from build123d import *

# Parameters (mm, degrees)
SKETCH011_R      = 1
EXTRUDE013_DEPTH = 8
SKETCH009_R      = 1.2
EXTRUDE012_DEPTH = 9.3
CHAMFER001_SIZE  = 0.15
SKETCH012_R      = 0.75
EXTRUDE014_DEPTH = 2
FILLET011_R      = 0.3


with BuildPart() as extrude013:
    # Sketch011 → Extrude013 (new body)
    with BuildSketch(Plane.XY.offset(9.3)):
        with Locations((-2.5, 0)):
            Circle(SKETCH011_R)
    extrude(amount=-EXTRUDE013_DEPTH)


with BuildPart() as pinfemale002:
    # Sketch009 → Extrude012 (new body)
    with BuildSketch(Plane.XY.offset(9.6)):
        with Locations((-2.5, 0)):
            Circle(SKETCH009_R)
    extrude(amount=-EXTRUDE012_DEPTH)


with BuildPart() as pinfemale002_1:
    # Extrude012 placement: moved
    add(pinfemale002.part.moved(Location((0, 0, -0.3))))

    # Cut007: cut Extrude013
    add(extrude013.part, mode=Mode.SUBTRACT)

    # Chamfer001
    chamfer001_edges = [pinfemale002_1.edges().sort_by_distance(p)[0] for p in [
        (-3.5, 0, 9.3),
    ]]
    chamfer(chamfer001_edges, length=CHAMFER001_SIZE)


with BuildPart() as pinfemale003:
    # Sketch012 → Extrude014 (new body)
    with BuildSketch(Plane(origin=(0, 0, 0), x_dir=(1, 0, 0), z_dir=(0, 0, -1))):
        with Locations((-2.5, 0)):
            Circle(SKETCH012_R)
    extrude(amount=EXTRUDE014_DEPTH)

    # Fillet011
    fillet011_edges = [pinfemale003.edges().sort_by_distance(p)[0] for p in [
        (-3.25, 0, -2),
    ]]
    fillet(fillet011_edges, radius=FILLET011_R)

    # Fusion006: union pinFemale002
    add(pinfemale002_1.part)


with BuildPart() as part_mirroring004:
    # Part__Mirroring004: instance of pinFemale003
    add(pinfemale003.part.mirror(Plane(origin=(0, 0, 0), x_dir=(0, -1, 0), z_dir=(1, 0, 0))))


solid = part_mirroring004.part
Geometry: final body of the model. Coordinates: model frame, mm. A direction names the side the tool comes from. Coordinates: 2 decimals unless noted, no trailing zeros. Loops run counter-clockwise (first coordinate to the right, second up) from the corner with the lowest first, then second, coordinate; pieces in that order, holes last. Notation, with made-up numbers: M 6,34.5 L 10,34.5 A9 cw 10,39.5 Z; hole C -32,21.5 d7. An arc over 180 degrees is marked long. One line per item, written item: value. Start each with the question number.
1) Draft query along Y for faces 1 (the flat face through (2.5, 0, -2)), 2 (the cylindrical face through (3.095, 0.456, -0.838)), 3 (the cylindrical face through (3.3, -0.6, 5.3)). Return one class per face: released by +Y, released by -Y, zero draft, split by the parting line, or undercut.
2) Cut plane C-C (z = 7). Return loops of the section in (x, y), then the cut area to 3 significant figures.
3) Cut plane B-B (x = 2.5). Return loops of the section in (y, z), then the cut area to 3 significant figures.
4) Material intervals for L1, parallel to Y at x = 2.5, z = 4; L2, parallel to X at y = -0.8, z = 7; L3, parallel to Z at x = 1.95, y = 0.7, sorted ascending. Write a range as from..to.
5) Cut plane A-A (y = 0). Return loops of the section in (x, z), then the cut area to 3 significant figures.
6) Reachability of faces 4 (the cylindrical face through (1.355, 0.36, 4.715)), 5 (the flat face through (3, 0, 1.3)) from +Z, -Z, +X, -X, +Y, -Y: full face, straight path, thin tool, end or side. Return the list, or none.
Evaluation:
1. face 1: zero draft
1. face 2: split by the parting line
1. face 3: undercut
2. outline: C 2.5,0 d2.4; hole C 2.5,0 d2
2. area: 1.38 mm^2
3. outline: M -1.2,0 L -0.75,0 L -0.75,-1.7 A0.3 ccw -0.45,-2 L 0.45,-2 A0.3 ccw 0.75,-1.7 L 0.75,0 L 1.2,0 L 1.2,9.3 L 1.15,9.3 L 1,9.15 L 1,1.3 L -1,1.3 L -1,9.15 L -1.15,9.3 L -1.2,9.3 Z
3. area: 9.26 mm^2
4. L1: -1.2..-1, 1..1.2
4. L2: 1.61..1.9, 3.1..3.39
4. L3: 0..1.3
5. outline: M 1.3,0 L 1.75,0 L 1.75,-1.7 A0.3 ccw 2.05,-2 L 2.95,-2 A0.3 ccw 3.25,-1.7 L 3.25,0 L 3.7,0 L 3.7,9.3 L 3.65,9.3 L 3.5,9.15 L 3.5,1.3 L 1.5,1.3 L 1.5,9.15 L 1.35,9.3 L 1.3,9.3 Z
5. area: 9.26 mm^2
6. face 4: +Z, -Z
6. face 5: +Z
